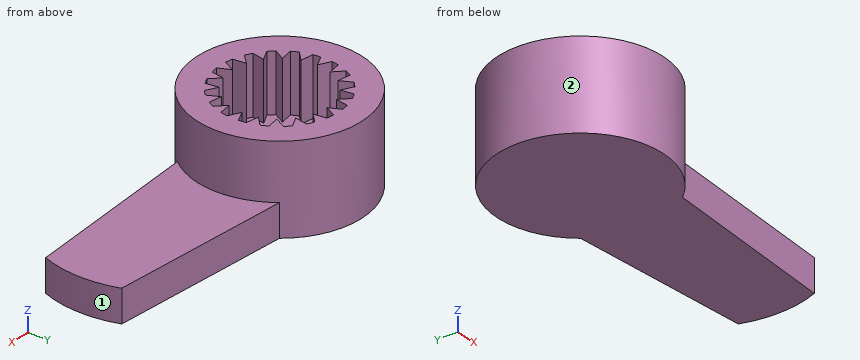
```python
from build123d import *

# Parameters (mm, degrees)
SKETCH2_R           = 3.55
BOSS_EXTRUDE1_DEPTH = 3.8
BOSS_EXTRUDE2_DEPTH = 1.4
SKETCH5_R           = 2.549999919
CUT_EXTRUDE1_DEPTH  = 2.5
BOSS_EXTRUDE3_DEPTH = 2.5


with BuildPart() as part:
    # Sketch2 → Boss-Extrude1 (new body)
    with BuildSketch(Plane.XY):
        Circle(SKETCH2_R)
    extrude(amount=-BOSS_EXTRUDE1_DEPTH)

    # Sketch4 → Boss-Extrude2 (add)
    with BuildSketch(Plane.XY.offset(-2.4)):
        with BuildLine():
            Line((2.776387215, 2.212277889), (10.622617722, 1.649999976))
            ThreePointArc((10.622617722, 1.649999976), (10.913548722, 0), (10.622617722, -1.649999976))
            Line((10.622617722, -1.649999976), (2.776387215, -2.212277889))
            ThreePointArc((2.776387215, -2.212277889), (3.549999952, 0), (2.776387215, 2.212277889))
        make_face()
    extrude(amount=-BOSS_EXTRUDE2_DEPTH)

    # Sketch5 → Cut-Extrude1 (cut)
    with BuildSketch(Plane.XY):
        Circle(SKETCH5_R)
    extrude(amount=-CUT_EXTRUDE1_DEPTH, mode=Mode.SUBTRACT)

    # Sketch3 → Boss-Extrude3 (add)
    with BuildSketch(Plane.XY):
        with BuildLine():
            Line((-0.244697916, 2.538232164), (0, 2.049999952))
            Line((0, 2.049999952), (0.244697916, 2.538232164))
            ThreePointArc((0.244697916, 2.538232164), (0, 2.549999919), (-0.244697916, 2.538232164))
        make_face()
        with BuildLine():
            Line((0.551635326, 2.489618054), (0.633484824, 1.949665813))
            Line((0.633484824, 1.949665813), (1.017078422, 2.338386424))
            ThreePointArc((1.017078422, 2.338386424), (0.787993311, 2.42519404), (0.551635326, 2.489618054))
        make_face()
        with BuildLine():
            Line((1.29397066, 2.197302783), (1.204959739, 1.6584848))
            Line((1.204959739, 1.6584848), (1.689900206, 1.90964313))
            ThreePointArc((1.689900206, 1.90964313), (1.498852346, 2.06299327), (1.29397066, 2.197302783))
        make_face()
        with BuildLine():
            Line((1.90964313, 1.689900206), (1.6584848, 1.204959739))
            Line((1.6584848, 1.204959739), (2.197302783, 1.29397066))
            ThreePointArc((2.197302783, 1.29397066), (2.06299327, 1.498852346), (1.90964313, 1.689900206))
        make_face()
        with BuildLine():
            Line((2.338386424, 1.017078422), (1.949665813, 0.633484824))
            Line((1.949665813, 0.633484824), (2.489618054, 0.551635326))
            ThreePointArc((2.489618054, 0.551635326), (2.42519404, 0.787993311), (2.338386424, 1.017078422))
        make_face()
        with BuildLine():
            Line((2.538232164, 0.244697916), (2.049999952, 0))
            Line((2.049999952, 0), (2.538232164, -0.244697916))
            ThreePointArc((2.538232164, -0.244697916), (2.549999919, 0), (2.538232164, 0.244697916))
        make_face()
        with BuildLine():
            Line((2.489618054, -0.551635326), (1.949665813, -0.633484824))
            Line((1.949665813, -0.633484824), (2.338386424, -1.017078422))
            ThreePointArc((2.338386424, -1.017078422), (2.42519404, -0.787993311), (2.489618054, -0.551635326))
        make_face()
        with BuildLine():
            Line((2.197302783, -1.29397066), (1.6584848, -1.204959739))
            Line((1.6584848, -1.204959739), (1.90964313, -1.689900206))
            ThreePointArc((1.90964313, -1.689900206), (2.06299327, -1.498852346), (2.197302783, -1.29397066))
        make_face()
        with BuildLine():
            Line((1.689900206, -1.90964313), (1.204959739, -1.6584848))
            Line((1.204959739, -1.6584848), (1.29397066, -2.197302783))
            ThreePointArc((1.29397066, -2.197302783), (1.498852346, -2.06299327), (1.689900206, -1.90964313))
        make_face()
        with BuildLine():
            Line((1.017078422, -2.338386424), (0.633484824, -1.949665813))
            Line((0.633484824, -1.949665813), (0.551635326, -2.489618054))
            ThreePointArc((0.551635326, -2.489618054), (0.787993311, -2.42519404), (1.017078422, -2.338386424))
        make_face()
        with BuildLine():
            Line((0.244697916, -2.538232164), (0, -2.049999952))
            Line((0, -2.049999952), (-0.244697916, -2.538232164))
            ThreePointArc((-0.244697916, -2.538232164), (0, -2.549999919), (0.244697916, -2.538232164))
        make_face()
        with BuildLine():
            Line((-0.551635326, -2.489618054), (-0.633484824, -1.949665813))
            Line((-0.633484824, -1.949665813), (-1.017078422, -2.338386424))
            ThreePointArc((-1.017078422, -2.338386424), (-0.787993311, -2.42519404), (-0.551635326, -2.489618054))
        make_face()
        with BuildLine():
            Line((-1.29397066, -2.197302783), (-1.204959739, -1.6584848))
            Line((-1.204959739, -1.6584848), (-1.689900206, -1.90964313))
            ThreePointArc((-1.689900206, -1.90964313), (-1.498852346, -2.06299327), (-1.29397066, -2.197302783))
        make_face()
        with BuildLine():
            Line((-1.90964313, -1.689900206), (-1.6584848, -1.204959739))
            Line((-1.6584848, -1.204959739), (-2.197302783, -1.29397066))
            ThreePointArc((-2.197302783, -1.29397066), (-2.06299327, -1.498852346), (-1.90964313, -1.689900206))
        make_face()
        with BuildLine():
            Line((-2.338386424, -1.017078422), (-1.949665813, -0.633484824))
            Line((-1.949665813, -0.633484824), (-2.489618054, -0.551635326))
            ThreePointArc((-2.489618054, -0.551635326), (-2.42519404, -0.787993311), (-2.338386424, -1.017078422))
        make_face()
        with BuildLine():
            Line((-2.538232164, -0.244697916), (-2.049999952, 0))
            Line((-2.049999952, 0), (-2.538232164, 0.244697916))
            ThreePointArc((-2.538232164, 0.244697916), (-2.549999919, 0), (-2.538232164, -0.244697916))
        make_face()
        with BuildLine():
            Line((-2.489618054, 0.551635326), (-1.949665813, 0.633484824))
            Line((-1.949665813, 0.633484824), (-2.338386424, 1.017078422))
            ThreePointArc((-2.338386424, 1.017078422), (-2.42519404, 0.787993311), (-2.489618054, 0.551635326))
        make_face()
        with BuildLine():
            Line((-2.197302783, 1.29397066), (-1.6584848, 1.204959739))
            Line((-1.6584848, 1.204959739), (-1.90964313, 1.689900206))
            ThreePointArc((-1.90964313, 1.689900206), (-2.06299327, 1.498852346), (-2.197302783, 1.29397066))
        make_face()
        with BuildLine():
            Line((-1.689900206, 1.90964313), (-1.204959739, 1.6584848))
            Line((-1.204959739, 1.6584848), (-1.29397066, 2.197302783))
            ThreePointArc((-1.29397066, 2.197302783), (-1.498852346, 2.06299327), (-1.689900206, 1.90964313))
        make_face()
        with BuildLine():
            Line((-1.017078422, 2.338386424), (-0.633484824, 1.949665813))
            Line((-0.633484824, 1.949665813), (-0.551635326, 2.489618054))
            ThreePointArc((-0.551635326, 2.489618054), (-0.787993311, 2.42519404), (-1.017078422, 2.338386424))
        make_face()
    extrude(amount=-BOSS_EXTRUDE3_DEPTH)


solid = part.part
```
Part model, mm, in its own coordinate system. Face numbers are marked on the shaded views. A direction names the side the tool comes from. Give positions to 0.01 mm unless a question says otherwise; leave off trailing zeros. Order: outer loops, then holes, each group sorted by start corner. A loop starts at its lowest first (then second) coordinate and runs counter-clockwise, first axis right, second up. Notation, with made-up numbers: M -32.75,63.5 L 10.25,63.5 A14 cw 10.25,69.5 Z; hole C -20,2.5 d4. An arc over 180 degrees is marked long. Use a Markdown table: item, result. Add a question column.
(1) 3-axis set-ups, long thin cutter, end or side, ignore diameter. For the marked faces 1 and 2: which of +Z, -Z, +X, -X, +Y, -Y reach the whole face in a straight line?
(2) Probe line 1 along Y through (x, z) = (1.75, -2.45); line 2 along Z through (x, y) = (-0.5, -0.25); line 3 along Z through (x, y) = (4.5, 1.25). List the from-to ranges inside material, lowest first. Write a range as [from, to].
(3) Saw through at B-B, the plane y = 1.5. Give the cut face in (x, z), and give its area (3 significant figures).
(4) Saw through at D-D, the plane x = -1.5. Give the cut face in (y, z).
(5) Drop flat-ended pins along their axis: P1, Ø1.3, axis at x = 7, y = 0, coming from the +Z side; P2, Ø1, axis at y = -2.5, z = -1, coming from the +X side; P3, Ø1, axis at y = 1, z = -3, coming from the +X side. Give the stop position or say it passes through.
(6) Saw through at C-C, the plane z = -2.9. Give the cut face in (x, y).
(7) Saw through at A-A, the plane x = 3. Give the cut face in (y, z), and give its area (3 significant figures).
Answer key:
| question | item | result |
|---|---|---|
| 1 | face 1 | +Z, -Z, +X |
| 1 | face 2 | +Z |
| 2 | line 1 | [-3.09, -1.85], [-1.38, -1.22], [1.22, 1.38], [1.85, 3.09] |
| 2 | line 2 | [-3.8, -2.5] |
| 2 | line 3 | [-3.8, -2.4] |
| 3 | outline | M -3.22,-3.8 L 10.67,-3.8 L 10.67,-2.4 L 3.22,-2.4 L 3.22,0 L 1.81,0 L 1.81,-2.5 L -1.81,-2.5 L -1.81,0 L -3.22,0 Z |
| 3 | area | 25.8 mm^2 |
| 4 | outline | M -3.22,-3.8 L 3.22,-3.8 L 3.22,0 L 1.81,0 L 1.81,-2.5 L -1.81,-2.5 L -1.81,0 L -3.22,0 Z |
| 5 | P1 | z = -2.4 |
| 5 | P2 | x = 2.93 |
| 5 | P3 | x = 10.89 |
| 6 | outline | M 2.78,-2.21 L 10.62,-1.65 A4.82 ccw 10.62,1.65 L 2.78,2.21 A3.55 ccw long Z |
| 7 | outline | M -2.2,-3.8 L 2.2,-3.8 L 2.2,-2.4 L 1.9,-2.4 L 1.9,0 L -1.9,0 L -1.9,-2.4 L -2.2,-2.4 Z |
| 7 | area | 15.3 mm^2 |
